from build123d import *

# Parameters (mm, degrees)
BOSS_EXTRUDE1_DEPTH = 100
BOSS_EXTRUDE2_START = 15
BOSS_EXTRUDE2_DEPTH = 15
SKETCH3_W           = 15
SKETCH3_H           = 15
BOSS_EXTRUDE3_DEPTH = 30
SKETCH4_W           = 15
SKETCH4_H           = 15
BOSS_EXTRUDE4_DEPTH = 10
SKETCH7_W           = 31
SKETCH7_H           = 40
CUT_EXTRUDE2_DEPTH  = 122.862627577
SKETCH8_W           = 15
SKETCH8_H           = 15
BOSS_EXTRUDE5_DEPTH = 39
SKETCH9_W           = 15
SKETCH9_H           = 15
BOSS_EXTRUDE6_DEPTH = 15
CUT_EXTRUDE4_DEPTH  = 145.762736918


with BuildPart() as part:
    # Sketch1 → Boss-Extrude1 (new body)
    with BuildSketch(Plane.XY):
        with BuildLine():
            Line((-10, 53.574714185), (-10, -5.425285815))
            ThreePointArc((-10, -5.425285815), (-7.071067812, -12.496353627), (0, -15.425285815))
            Line((0, -15.425285815), (20, -15.425285815))
            Line((20, -15.425285815), (20, -30.425285815))
            Line((20, -30.425285815), (-20, -30.425285815))
            Line((-20, -30.425285815), (-20, -50.697633081))
            ThreePointArc((-20, -50.697633081), (-54.251088478, 5.202826051), (-10, 53.574714185))
        make_face()
    extrude(amount=-BOSS_EXTRUDE1_DEPTH)

    # Sketch2 → Boss-Extrude2 (add)
    with BuildSketch(Plane.XY.offset(BOSS_EXTRUDE2_START)):
        with BuildLine():
            Line((20, -25.425285815), (20, -30.425285815))
            Line((20, -30.425285815), (-20, -30.425285815))
            Line((-20, -30.425285815), (-20, -50.697633081))
            ThreePointArc((-20, -50.697633081), (-42.112075999, -34.595130511), (-53.615715713, -9.777782398))
            Line((-53.615715713, -9.777782398), (20, -25.425285815))
        make_face()
    extrude(amount=-BOSS_EXTRUDE2_DEPTH)

    # Sketch3 → Boss-Extrude3 (add)
    with BuildSketch(Plane.XY):
        with Locations((-12.5, 31.074714185)):
            Rectangle(SKETCH3_W, SKETCH3_H)
    extrude(amount=-BOSS_EXTRUDE3_DEPTH)

    # Sketch4 → Boss-Extrude4 (add)
    with BuildSketch(Plane.XY):
        with Locations((-12.5, 31.074714185)):
            Rectangle(SKETCH4_W, SKETCH4_H)
    extrude(amount=BOSS_EXTRUDE4_DEPTH)

    # Sketch7 → Cut-Extrude2 (cut, through all)
    with BuildSketch(Plane(origin=(-10, 0, 0), x_dir=(0, 0, -1), z_dir=(1, 0, 0))):
        with Locations((45.5, 33.574714185)):
            Rectangle(SKETCH7_W, SKETCH7_H)
    extrude(amount=-CUT_EXTRUDE2_DEPTH, mode=Mode.SUBTRACT)

    # Sketch8 → Boss-Extrude5 (add)
    with BuildSketch(Plane(origin=(0, 0, -100), x_dir=(-1, 0, 0), z_dir=(0, 0, -1))):
        with Locations((12.5, 31.074714185)):
            Rectangle(SKETCH8_W, SKETCH8_H)
    extrude(amount=-BOSS_EXTRUDE5_DEPTH)

    # Sketch9 → Boss-Extrude6 (add)
    with BuildSketch(Plane(origin=(0, 0, -100), x_dir=(-1, 0, 0), z_dir=(0, 0, -1))):
        with Locations((12.5, 31.074714185)):
            Rectangle(SKETCH9_W, SKETCH9_H)
    extrude(amount=BOSS_EXTRUDE6_DEPTH)

    # Sketch10 → Cut-Extrude4 (cut, through all)
    with BuildSketch(Plane(origin=(0, -15.425285815, 0), x_dir=(1, 0, 0), z_dir=(0, 1, 0))):
        with BuildLine():
            Line((5, 10), (5, 90))
            ThreePointArc((5, 90), (10, 95), (15, 90))
            Line((15, 90), (15, 10))
            ThreePointArc((15, 10), (10, 5), (5, 10))
        make_face()
    extrude(amount=-CUT_EXTRUDE4_DEPTH, mode=Mode.SUBTRACT)


solid = part.part
CAD build for the part. Positions are in the model's coordinates, mm. A direction names the side the tool comes from. Coordinates: 2 decimals unless noted, no trailing zeros. Order: outer loops, then holes, each group sorted by start corner. A loop starts at its lowest first (then second) coordinate and runs counter-clockwise, first axis right, second up. Notation, with made-up numbers: (87.25, -17) -> (103.25, -17) arc R13 ccw to (103.25, -9) -> close; hole circle Ø3 at (-11, 49.25). An arc over 180 degrees is marked (long way). Answer in a Markdown table with one row per item.
1) Drill centre lines: line 1 (Z direction, x = -33.5, y = 31.5); line 2 (Z direction, x = -35, y = 12); line 3 (Z direction, x = -41, y = -23). Where is each one in solid material? Low to high.
Check values:
| item | result |
|---|---|
| line 1 | -100 to -61, -30 to 0 |
| line 2 | -100 to 0 |
| line 3 | -100 to 15 |
2) Mould opens along Z. For faces 1 (the face through (-4, -30.425, -42)), 2 (the face through (5, -23, -49)), 3 (the face through (-12, 31, -115)), 4 (the face through (-31, 13.575, -45)) say: pulls with the +Z half, pulls with the -Z half, needs draft (parallel to the pull), parting line crosses it, or undercut.
Check values:
| item | result |
|---|---|
| face 1 | needs draft |
| face 2 | undercut |
| face 3 | pulls with the -Z half |
| face 4 | undercut |
3) Band-saw the part on B-B (x = 10). List the corners of the cut face in (y, z), and give its area (3 significant figures).
Check values:
| item | result |
|---|---|
| outline | (-30.43, -100) -> (-15.43, -100) -> (-15.43, -95) -> (-30.43, -95) -> close; (-30.43, -5) -> (-15.43, -5) -> (-15.43, 0) -> (-23.3, 0) -> (-23.3, 15) -> (-30.43, 15) -> close |
| area | 257 mm2 |
4) Which spindle directions (+Z, -Z, +X, -X, +Y, -Y) get a long thin tool onto all of the face, cutting with end or side? Do faces 5 (the face through (-9, 23.575, -6)), 6 (the face through (-9, 38.575, -6)), 7 (the face through (-10, 9, -49)), 8 (the face through (-10, 46, -15)). Say none if no direction does.
Check values:
| item | result |
|---|---|
| face 5 | +Z, +X |
| face 6 | +Z, +X, +Y |
| face 7 | +Z, -Z, +X |
| face 8 | +Z, -Z, +X, +Y |
5) Flat gauge pins, fed straight in: P1, Ø8.5, axis at y = 11, z = -65, coming from the +X side; P2, Ø16.5, axis at x = -10.5, z = -90, coming from the -Y side; P3, Ø16, axis at x = 9, z = -50, coming from the +Y side; P4, Ø2, axis at x = -18.5, y = -37, coming from the +Z side. Where does each tip first touch, or does it go through?
Check values:
| item | result |
|---|---|
| P1 | x = -10 |
| P2 | y = -30.43 |
| P3 | y = -15.43 |
| P4 | through |
6) Band-saw the part on A-A (z = -58). List the corners of the cut face in (x, y).
Check values:
| item | result |
|---|---|
| outline | (-52.78, 13.57) arc R54.5 ccw to (-20, -50.7) -> (-20, -30.43) -> (5, -30.43) -> (5, -15.43) -> (0, -15.43) arc R10 cw to (-10, -5.43) -> (-10, 13.57) -> close; (15, -30.43) -> (20, -30.43) -> (20, -15.43) -> (15, -15.43) -> close |
7) Band-saw the part on D-D (x = -7.5). List the corners of the cut face in (y, z), and give its area (3 significant figures).
Check values:
| item | result |
|---|---|
| outline | (-30.43, -100) -> (-12.04, -100) -> (-12.04, 0) -> (-19.58, 0) -> (-19.58, 15) -> (-30.43, 15) -> close; (23.57, -115) -> (38.57, -115) -> (38.57, -61) -> (23.57, -61) -> close; (23.57, -30) -> (38.57, -30) -> (38.57, 10) -> (23.57, 10) -> close |
| area | 3,410 mm2 |
8) Band-saw the part on C-C (y = 27). List the corners of the cut face in (x, z), and give its area (3 significant figures).
Check values:
| item | result |
|---|---|
| outline | (-47.34, -100) -> (-20, -100) -> (-20, -115) -> (-5, -115) -> (-5, -61) -> (-47.34, -61) -> close; (-47.34, -30) -> (-5, -30) -> (-5, 10) -> (-20, 10) -> (-20, 0) -> (-47.34, 0) -> close |
| area | 3,300 mm2 |
